Geometry: final body of the model. Coordinates: model frame, mm. Face numbers are marked on the shaded views. A direction names the side the tool comes from. Coordinates: 2 decimals unless noted, no trailing zeros. Write each loop counter-clockwise with the first axis right and the second up, starting at its lowest first coordinate (ties: lowest second). Pieces come first, ordered by that corner, then holes. Notation, with made-up numbers: M 41.25,2 L 53.25,2 A19 cw 53.25,29 Z; hole C 21.25,80.5 d6. An arc over 180 degrees is marked long. Write item = value, one per line. Start each with the question number.
Item 1: Pull-direction query (Y, two-part tool) for the marked faces 3, 4 and 5; classes: +Y half, -Y half, draft (parallel to the pull), parting line (faces both ways), or undercut.
Item 2: Ray query, L1, parallel to X at y = -65, z = 27; L2, parallel to Y at x = 74, z = 18. Return the intervals inside material, ascending. Write a range as [from, to].
Item 3: Section B-B on y = -47. Output: boundary loops of the cut face in (x, z), plus the area to 3 significant figures.
Item 4: Section A-A on z = 18.5. Output: boundary loops of the cut face in (x, y).
Item 5: Reachability of the marked faces 1 and 2 from +Z, -Z, +X, -X, +Y, -Y: full face, straight path, thin tool, end or side. Return the list, or none.
Item 6: Section C-C on x = 97.5. Output: boundary loops of the cut face in (y, z), plus the area to 3 significant figures.
from build123d import *

# Parameters (mm, degrees)
F0_W     = 121.05
F0_H     = 79.05
F1_DEPTH = 2.5
F0_W_2   = 126.05
F0_H_2   = 84.05
F2_DEPTH = 37


with BuildPart() as f1:
    # F0 (on Top) → F1 (new body)
    with BuildSketch(Plane.XY):
        with Locations((63.025, -42.025)):
            Rectangle(F0_W, F0_H)
        Polygon((8.15, -78.55), (8.15, -5.5), (20.95, -5.5), (20.95, -3.5), (23.45, -3.5), (23.45, -5.5), (48.15, -5.5), (48.15, -3.5), (50.65, -3.5), (50.65, -5.5), (75.4, -5.5), (75.4, -3.5), (77.9, -3.5), (77.9, -5.5), (102.6, -5.5), (102.6, -3.5), (105.1, -3.5), (105.1, -5.5), (117.9, -5.5), (117.9, -78.55), (105.1, -78.55), (105.1, -80.55), (102.6, -80.55), (102.6, -78.55), (77.9, -78.55), (77.9, -80.55), (75.4, -80.55), (75.4, -78.55), (50.65, -78.55), (50.65, -80.55), (48.15, -80.55), (48.15, -78.55), (23.45, -78.55), (23.45, -80.55), (20.95, -80.55), (20.95, -78.55), align=None, mode=Mode.SUBTRACT)
    extrude(amount=F1_DEPTH)

    # F0 (on Top) → F2 (join)
    with BuildSketch(Plane.XY):
        with Locations((63.025, -42.025)):
            Rectangle(F0_W_2, F0_H_2)
        with Locations((63.025, -42.025)):
            Rectangle(F0_W, F0_H, mode=Mode.SUBTRACT)
    extrude(amount=F2_DEPTH)


solid = f1.part
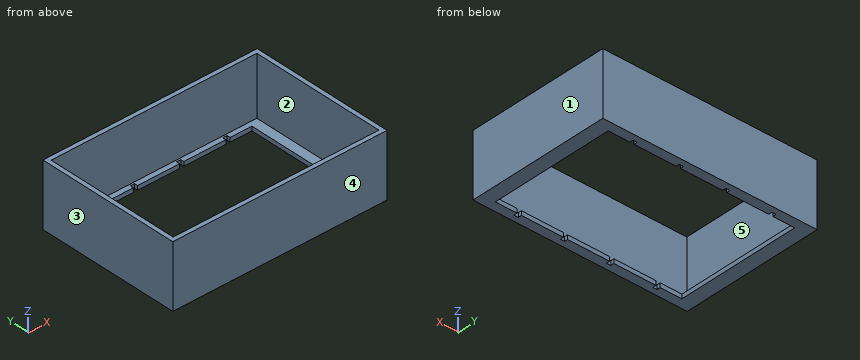
Responses:
q1.face_3 = draft
q1.face_4 = -Y half
q1.face_5 = undercut
q2.L1 = [0, 2.5], [123.55, 126.05]
q2.L2 = [-84.05, -81.55], [-2.5, 0]
q3.outline = M 0,0 L 8.15,0 L 8.15,2.5 L 2.5,2.5 L 2.5,37 L 0,37 Z; M 117.9,0 L 126.05,0 L 126.05,37 L 123.55,37 L 123.55,2.5 L 117.9,2.5 Z
q3.area = 213 mm²
q4.outline = M 0,-84.05 L 126.05,-84.05 L 126.05,0 L 0,0 Z; hole M 2.5,-81.55 L 123.55,-81.55 L 123.55,-2.5 L 2.5,-2.5 Z
q5.face_1 = +Z, -Z, +X, +Y, -Y
q5.face_2 = +Z
q6.outline = M -84.05,0 L -78.55,0 L -78.55,2.5 L -81.55,2.5 L -81.55,37 L -84.05,37 Z; M -5.5,0 L 0,0 L 0,37 L -2.5,37 L -2.5,2.5 L -5.5,2.5 Z
q6.area = 200 mm²
